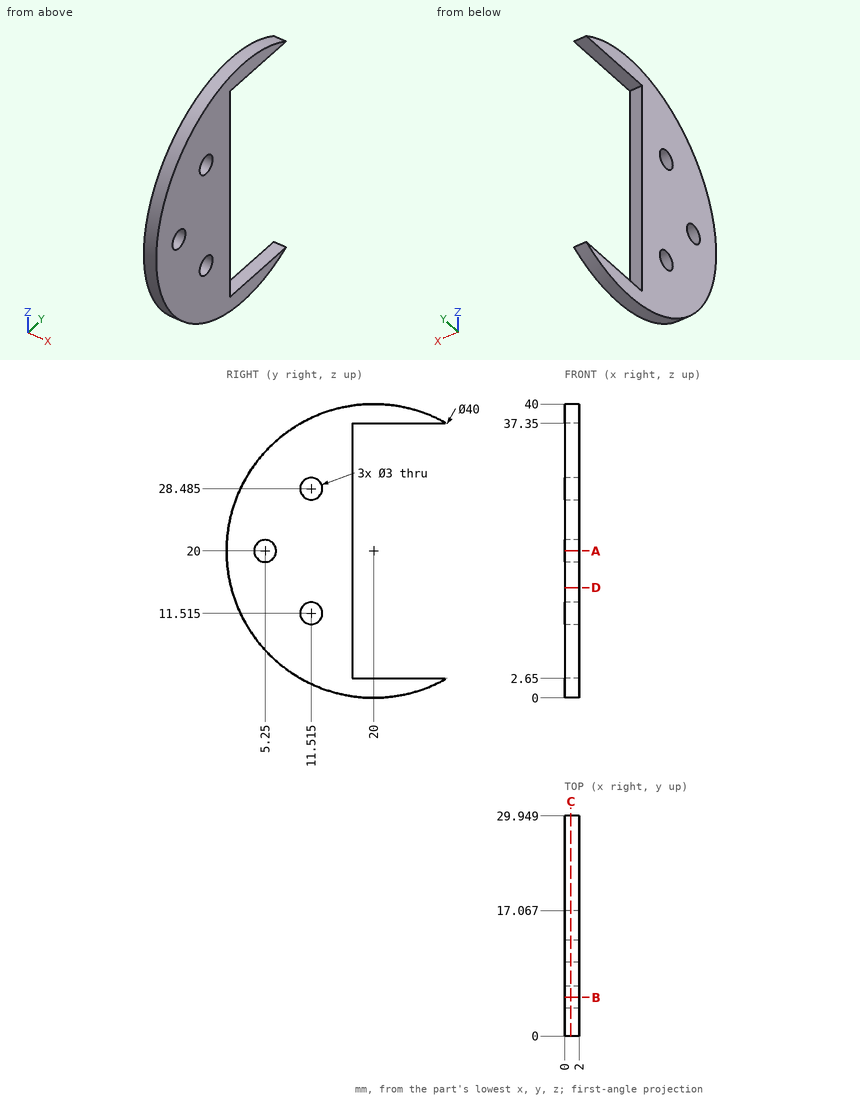
Print and shaded views of the part. All mm, measured from the part's lowest x, y and z. Round coordinates to 2 decimals unless told otherwise and drop trailing zeros. Write each loop counter-clockwise with the first axis right and the second up, starting at its lowest first coordinate (ties: lowest second). Pieces come first, ordered by that corner, then holes. Notation, with made-up numbers: (4.5, -10.75) - (32.5, -10.75) arc R18 ccw to (32.5, 8.25) - close; hole circle Ø2 at (31.25, -17.75). An arc over 180 degrees is marked (long way). Use CSV: the item, a comma, the result in double quotes. Start each with the question number.
Item 1: Drill centre lines: L1, parallel to Y at x = 0.5, z = 20; L2, parallel to Z at x = 0.9, y = 10.5; L3, parallel to Z at x = 1.4, y = 19.5. Where is each one in solid material? Low to high. Write a range as [from, to].
Item 2: Band-saw the part on A-A (z = 20). Write the cut outline in (x, y).
Item 3: Band-saw the part on D-D (z = 15). Write the cut outline in (x, y) (1 decimal).
Item 4: Band-saw the part on C-C (x = 0.85). State how many separate pieces and enclosed holes the cut face has, and give its area (3 significant figures).
Item 5: Pin check, flat tips, straight feed: P1, Ø1, axis at x = 1.5, y = 21, coming from the +Z side; P2, Ø1, axis at x = 1.5, y = 25, coming from the -Z side; P3, Ø5, axis at y = 19.5, z = 9.5, coming from the -X side; P4, Ø1, axis at x = 1.5, y = 4.5, coming from the +Z side. Stop position of each tip, or through.
Item 6: Band-saw the part on B-B (y = 5.25). Write the cut outline in (x, z).
Checked values:
1,L1,"y = [0, 3.75], [6.75, 17.07]"
1,L2,"z = [2.4, 10.41], [12.62, 27.38], [29.59, 37.6]"
1,L3,"z = [0.01, 2.65], [37.35, 39.99]"
2,outline,"(0, 0) - (2, 0) - (2, 3.75) - (0, 3.75) - close; (0, 6.75) - (2, 6.75) - (2, 17.07) - (0, 17.07) - close"
3,outline,"(0, 0.6) - (2, 0.6) - (2, 17.1) - (0, 17.1) - close"
4,separate pieces,"1"
4,enclosed holes,"3"
4,area,"541 mm²"
5,P1,"stops at z = 39.99"
5,P2,"stops at z = 0.51"
5,P3,"stops at x = 0"
5,P4,"stops at z = 33.23"
6,outline,"(0, 6.49) - (2, 6.49) - (2, 18.5) - (0, 18.5) - close; (0, 21.5) - (2, 21.5) - (2, 33.51) - (0, 33.51) - close"
